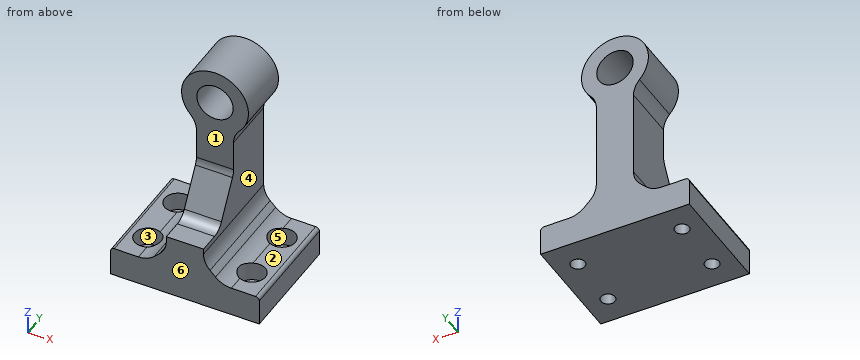
```python
from build123d import *

# Parameters (mm, degrees)
F0_R          = 6.223
F1_DEPTH      = 19.05
F2_SIZE       = 6.35
F4_R          = 7.62
F3_R          = 2.413
F5_DEPTH      = 73.661
F6_R          = 4.572
F7_DEPTH      = 6.35
F7_DEPTH_BACK = 63.501
F8_R          = 1.27
F10_DEPTH     = 25.4
F11_R         = 5.08


# Not quite as in the source:
# - a pattern or mirror of a feature is missing from the dataset's text; its kind, count and spacing are read off the source's solid


with BuildPart() as f1:
    # F0 (on Front) → F1 (new body, symmetric)
    with BuildSketch(Plane.XZ):
        with BuildLine():
            Line((-25.4, 10.16), (-25.4, 0))
            Line((-25.4, 0), (25.4, 0))
            Line((25.4, 0), (25.4, 10.16))
            Line((25.4, 10.16), (6.35, 10.16))
            Line((6.35, 10.16), (6.35, 52.7261902376))
            ThreePointArc((6.35, 52.7261902376), (0, 73.66), (-6.35, 52.7261902376))
            Line((-6.35, 52.7261902376), (-6.35, 10.16))
            Line((-6.35, 10.16), (-25.4, 10.16))
        make_face()
        with Locations((0, 62.23)):
            Circle(F0_R, mode=Mode.SUBTRACT)
    extrude(amount=F1_DEPTH, both=True)

    # F2
    f2_edges = [f1.edges().sort_by_distance(p)[0] for p in [
        (-6.35, 0, 10.16),
        (6.35, 0, 10.16),
    ]]
    chamfer(f2_edges, length=F2_SIZE)

    # F4
    f4_edges = [f1.edges().sort_by_distance(p)[0] for p in [
        (-6.35, 0, 52.72619),
        (-6.35, 0, 16.51),
        (-12.7, 0, 10.16),
        (12.7, 0, 10.16),
        (6.35, 0, 16.51),
        (6.35, 0, 52.72619),
    ]]
    fillet(f4_edges, radius=F4_R)

    # F3 (on face) → F5 (cut, through all)
    with BuildSketch(Plane(origin=(0, 0, 0), x_dir=(1, 0, 0), z_dir=(0, 0, -1))):
        with Locations((-17.78, 9.525)):
            Circle(F3_R)
        with Locations((-17.78, -9.525)):
            Circle(F3_R)
    f5 = extrude(amount=-F5_DEPTH, mode=Mode.SUBTRACT)

    # F5_copies: F5 across plane
    add(f5.mirror(Plane(origin=(0, 0, 0), x_dir=(0, 0, 1), z_dir=(1, 0, 0))), mode=Mode.SUBTRACT)

    # F6 (on face) → F7 (cut, two sides)
    with BuildSketch(Plane.XY.offset(10.16)) as f7_sk:
        with Locations((-17.78, 9.525)):
            Circle(F6_R)
        with Locations((-17.78, -9.525)):
            Circle(F6_R)
    f7 = extrude(amount=-F7_DEPTH, mode=Mode.SUBTRACT) + extrude(f7_sk.sketch, amount=F7_DEPTH_BACK, mode=Mode.SUBTRACT)

    # F7_copies: F7 across plane
    add(f7.mirror(Plane(origin=(2e-06, 0, 0), x_dir=(0, 0, 1), z_dir=(1, 0, 0))), mode=Mode.SUBTRACT)

    # F8
    f8_edges = [f1.edges().sort_by_distance(p)[0] for p in [
        (-25.4, 0, 10.16),
        (25.4, 0, 10.16),
    ]]
    fillet(f8_edges, radius=F8_R)

    # F9 (on Right) → F10 (cut, symmetric)
    with BuildSketch(Plane.YZ):
        Polygon((0, 37.4132022262), (0, 76.8906995654), (-23.6530974507, 76.8906995654), (-23.6530974507, 21.59), (-9.1355300647, 21.59), align=None)
    extrude(amount=F10_DEPTH, both=True, mode=Mode.SUBTRACT)

    # F11
    f11_edges = [f1.edges().sort_by_distance(p)[0] for p in [
        (0, 0, 37.413202),
        (0, -9.13553, 21.59),
    ]]
    fillet(f11_edges, radius=F11_R)


solid = f1.part
```
Could you check a few things on this model? Use its own coordinates, in mm. Face numbers are marked on the shaded views. A direction names the side the tool comes from. Round coordinates to 2 decimals unless told otherwise and drop trailing zeros. Write each loop counter-clockwise with the first axis right and the second up, starting at its lowest first coordinate (ties: lowest second). Pieces come first, ordered by that corner, then holes. Notation, with made-up numbers: M -19,23 L 26,23 A28 cw 26,47 Z; hole C 11.25,-13.5 d4. An arc over 180 degrees is marked long. Answer in a Markdown table with one row per item. Add a question column.
Q1. Imagine slicing it at A-A (z = 62.23). Please give me the cut outline in (x, y).
Q2. On a 3-axis mill with a long thin cutter (end or side, diameter ignored), from which of +Z, -Z, +X, -X, +Y, -Y can I reach the whole of each face in a straight line? I mean the marked faces 1, 2 and 3. Say none if no direction works.
Q3. Imagine slicing it at C-C (x = 0). Please give me the cut outline in (y, z).
Q4. If we mould it in two halves opening along Y, with no side actions, what happens to the marked faces 4, 5 and 6? For each: +Y half, -Y half, draft (parallel to the pull), parting line (faces both ways), or undercut.
Q5. Will these pins go through, and if not, where does the flat tip stop? pin 1 Ø7.5 at (x, y) = (-17.78, -9.525) entering from +Z; pin 2 Ø7.5 at (x, y) = (16.5, -8) entering from +Z; pin 3 Ø18.5 at (x, z) = (-3.5, 58.5) entering from -Y; pin 4 Ø1 at (x, z) = (-7, 36.5) entering from -Y.
Q6. Imagine slicing it at B-B (x = 17.78). Please give me the cut outline in (y, z).
Q7. Imagine slicing it at D-D (y = 17). Please give me the cut outline in (x, z), then the cut area to 3 significant figures.
Q8. If I drill on line 1 (Z direction, x = 0, y = 12); line 2 (Y direction, x = -21, z = 6.5); line 3 (Y direction, x = -17.78, z = 1.35), over which ranges is the centre line in solid material (lowest first)? Write a range as from..to.
Values:
| question | item | result |
|---|---|---|
| 1 | outline | M -11.43,0 L -6.22,0 L -6.22,19.05 L -11.43,19.05 Z; M 6.22,0 L 11.43,0 L 11.43,19.05 L 6.22,19.05 Z |
| 2 | face 1 | +Z, +X, -X, -Y |
| 2 | face 2 | +Z, +X, +Y, -Y |
| 2 | face 3 | +Z |
| 3 | outline | M -19.05,0 L 19.05,0 L 19.05,56.01 L 0,56.01 L 0,38.77 A5.08 cw -0.68,36.23 L -7.67,24.13 A5.08 cw -12.07,21.59 L -19.05,21.59 Z; M 0,68.45 L 19.05,68.45 L 19.05,73.66 L 0,73.66 Z |
| 4 | face 4 | draft |
| 4 | face 5 | undercut |
| 4 | face 6 | -Y half |
| 5 | pin 1 | z = 3.81 |
| 5 | pin 2 | z = 10.82 |
| 5 | pin 3 | y = 0 |
| 5 | pin 4 | through |
| 6 | outline | M -19.05,0 L -11.94,0 L -11.94,3.81 L -14.1,3.81 L -14.1,10.16 L -19.05,10.16 Z; M -7.11,0 L 7.11,0 L 7.11,3.81 L 4.95,3.81 L 4.95,10.16 L -4.95,10.16 L -4.95,3.81 L -7.11,3.81 Z; M 11.94,0 L 19.05,0 L 19.05,10.16 L 14.1,10.16 L 14.1,3.81 L 11.94,3.81 Z |
| 7 | outline | M -25.4,0 L 25.4,0 L 25.4,8.89 A1.27 ccw 24.13,10.16 L 15.86,10.16 A7.62 cw 10.47,12.39 L 8.58,14.28 A7.62 cw 6.35,19.67 L 6.35,49.28 A7.62 cw 8.38,54.46 A11.43 ccw long -8.38,54.46 A7.62 cw -6.35,49.28 L -6.35,19.67 A7.62 cw -8.58,14.28 L -10.47,12.39 A7.62 cw -15.86,10.16 L -24.13,10.16 A1.27 ccw -25.4,8.89 Z; hole C 0,62.23 d12.45 |
| 7 | area | 1,380 mm^2 |
| 8 | line 1 | 0..56.01, 68.45..73.66 |
| 8 | line 2 | -19.05..-12.77, -6.28..6.28, 12.77..19.05 |
| 8 | line 3 | -19.05..-11.94, -7.11..7.11, 11.94..19.05 |
